For this review, take the finished solid that the model builds, in its own axes (mm). A direction names the side the tool comes from. Round coordinates to 2 decimals unless told otherwise and drop trailing zeros. Loops run counter-clockwise (first coordinate to the right, second up) from the corner with the lowest first, then second, coordinate; pieces in that order, holes last.
1. Consider section B-B on z = 0. State the section outline as (x, y) points, then the cut area to 3 significant figures.
2. To check wall thickness, follow line 1 along X through (y, z) = (4.05, 0); line 2 along X through (y, z) = (2.85, 0); line 3 along Z through (x, y) = (-61.5, 3.2). State the ranges of each line that lie inside material, in increasing order.
3. Clearance check with a flat-ended pin moving along its axis: pin 1 Ø3.5 at (x, z) = (40, 0) entering from +Y. State where the tip first meets the part, or that it passes through.
4. Tool access review of faces 5 (the flat face through (-1, 0, -2)), 6 (the cylindrical face through (-55.277, 4.521, -0.309)): name each direction out of +Z, -Z, +X, -X, +Y, -Y from which nothing blocks a thin tool from reaching the whole face with its end or side.
5. Consider section A-A on x = 40. State the section outline as (y, z) points.
6. Draft analysis for pull direction Z (two halves, no side actions). For faces 1 (the cylindrical face through (-68, 3, 0)), 2 (the cylindrical face through (-62.17, 1.48, -0.44)), 3 (the cylindrical face through (38, 3, 0)), 4 (the flat face through (1, 3, -8)), state which applies: released by +Z, released by -Z, zero draft, split by the parting line, or undercut.
from build123d import *

# Parameters (mm, degrees)
SKETCH1_R           = 3
SKETCH1_R_2         = 2
BOSS_EXTRUDE1_DEPTH = 6
SKETCH3_R           = 4
CUT_EXTRUDE1_DEPTH  = 3


with BuildPart() as part:
    # Sketch1 → Boss-Extrude1 (new body)
    with BuildSketch(Plane(origin=(0, 0, 0), x_dir=(1, 0, 0), z_dir=(0, 1, 0))):
        with BuildLine():
            Line((-60, -8), (60, -8))
            ThreePointArc((60, -8), (68, 0), (60, 8))
            Line((60, 8), (-60, 8))
            ThreePointArc((-60, 8), (-68, 0), (-60, -8))
        make_face()
        with Locations(Location((-59.243309237, -0.211557176, 0), (0, 0, 270))):
            Circle(SKETCH1_R, mode=Mode.SUBTRACT)
        with Locations(Location((60, 0, 0), (0, 0, 270))):
            Circle(SKETCH1_R_2, mode=Mode.SUBTRACT)
        with Locations(Location((20, 0, 0), (0, 0, 270))):
            Circle(SKETCH1_R_2, mode=Mode.SUBTRACT)
        with Locations(Location((40, 0, 0), (0, 0, 270))):
            Circle(SKETCH1_R_2, mode=Mode.SUBTRACT)
        with Locations(Location((0, 0, 0), (0, 0, 270))):
            Circle(SKETCH1_R_2, mode=Mode.SUBTRACT)
    extrude(amount=BOSS_EXTRUDE1_DEPTH)

    # Sketch3 → Cut-Extrude1 (cut)
    with BuildSketch(Plane(origin=(0, 6, 0), x_dir=(1, 0, 0), z_dir=(0, 1, 0))):
        with Locations(Location((-59.243309237, -0.211557176, 0), (0, 0, 270))):
            Circle(SKETCH3_R)
    extrude(amount=-CUT_EXTRUDE1_DEPTH, mode=Mode.SUBTRACT)


solid = part.part
Resolved:
1. outline: (-68, 0) - (-62.24, 0) - (-62.24, 3) - (-63.24, 3) - (-63.24, 6) - (-68, 6) - close; (-56.25, 0) - (-2, 0) - (-2, 6) - (-55.25, 6) - (-55.25, 3) - (-56.25, 3) - close; (2, 0) - (18, 0) - (18, 6) - (2, 6) - close; (22, 0) - (38, 0) - (38, 6) - (22, 6) - close; (42, 0) - (58, 0) - (58, 6) - (42, 6) - close; (62, 0) - (68, 0) - (68, 6) - (62, 6) - close
1. area: 678 mm2
2. line 1: x = -68 to -63.24, -55.25 to -2, 2 to 18, 22 to 38, 42 to 58, 62 to 68
2. line 2: x = -68 to -62.24, -56.25 to -2, 2 to 18, 22 to 38, 42 to 58, 62 to 68
2. line 3: z = -7.86 to -3.09, 3.51 to 7.86
3. pin 1: passes through
4. face 5: +Z, -Z, +X, -X, -Y
4. face 6: +Y
5. outline: (0, -8) - (6, -8) - (6, -2) - (0, -2) - close; (0, 2) - (6, 2) - (6, 8) - (0, 8) - close
6. face 1: split by the parting line
6. face 2: undercut
6. face 3: undercut
6. face 4: released by -Z
